```python
from build123d import *

# Parameters (mm, degrees)
SKETCH_1_W            = 101.6
SKETCH_1_H            = 101.6
EXTRUDE_1_DEPTH       = 2.9718
CUT_EXTRUDE_1_DEPTH   = 144.714827333
MIRROR_2_COPY_1_DEPTH = 144.714827333
CUT_EXTRUDE_3_DEPTH   = 144.714827333


with BuildPart() as part:
    # 草图1 → 凸台-拉伸1 (new body)
    with BuildSketch(Plane(origin=(0, 0, 0), x_dir=(1, 0, 0), z_dir=(0, 1, 0))):
        with Locations((50.8, 50.8)):
            Rectangle(SKETCH_1_W, SKETCH_1_H)
    extrude(amount=EXTRUDE_1_DEPTH)

    # 草图1<3> → 切除-拉伸1 (cut, through all)
    with BuildSketch(Plane(origin=(0, 0, 0), x_dir=(1, 0, 0), z_dir=(0, 1, 0))):
        Polygon((37.676666667, 98.6282), (37.676666667, 101.6), (30.056666667, 101.6), (30.056666667, 98.6282), (31.866666667, 98.6282), (31.866666667, 93.6282), (29.866666667, 93.6282), (29.866666667, 90.6282), (31.866666667, 90.6282), (31.866666667, 86.6282), (35.866666667, 86.6282), (35.866666667, 90.6282), (37.866666667, 90.6282), (37.866666667, 93.6282), (35.866666667, 93.6282), (35.866666667, 98.6282), align=None)
    cut_extrude_1 = extrude(amount=CUT_EXTRUDE_1_DEPTH, mode=Mode.SUBTRACT)

    # 镜向1: 切除-拉伸1 across plane
    add(cut_extrude_1.mirror(Plane(origin=(0, 0, -50.8), x_dir=(1, 0, 0), z_dir=(0, 0, -1))), mode=Mode.SUBTRACT)

    # 镜向2: 切除-拉伸1 across plane
    add(cut_extrude_1.mirror(Plane(origin=(50.8, 0, 0), x_dir=(0, 0, 1), z_dir=(1, 0, 0))), mode=Mode.SUBTRACT)

    # 镜向2 copy 1 sketch → 镜向2 copy 1 (cut, through all)
    with BuildSketch(Plane(origin=(101.6, 0, -101.6), x_dir=(-1, 0, 0), z_dir=(0, 1, 0))):
        Polygon((37.676666667, 98.6282), (37.676666667, 101.6), (30.056666667, 101.6), (30.056666667, 98.6282), (31.866666667, 98.6282), (31.866666667, 93.6282), (29.866666667, 93.6282), (29.866666667, 90.6282), (31.866666667, 90.6282), (31.866666667, 86.6282), (35.866666667, 86.6282), (35.866666667, 90.6282), (37.866666667, 90.6282), (37.866666667, 93.6282), (35.866666667, 93.6282), (35.866666667, 98.6282), align=None)
    extrude(amount=MIRROR_2_COPY_1_DEPTH, mode=Mode.SUBTRACT)

    # 草图1<4> → 切除-拉伸3 (cut, through all)
    with BuildSketch(Plane(origin=(0, 0, 0), x_dir=(1, 0, 0), z_dir=(0, 1, 0))):
        Polygon((0, 71.543333333), (0, 63.923333333), (2.9718, 63.923333333), (2.9718, 65.733333333), (7.9718, 65.733333333), (7.9718, 63.733333333), (10.9718, 63.733333333), (10.9718, 65.733333333), (14.9718, 65.733333333), (14.9718, 69.733333333), (10.9718, 69.733333333), (10.9718, 71.733333333), (7.9718, 71.733333333), (7.9718, 69.733333333), (2.9718, 69.733333333), (2.9718, 71.543333333), align=None)
    cut_extrude_3 = extrude(amount=CUT_EXTRUDE_3_DEPTH, mode=Mode.SUBTRACT)

    # 镜向3: 切除-拉伸3 across plane
    add(cut_extrude_3.mirror(Plane(origin=(0, 0, -50.8), x_dir=(1, 0, 0), z_dir=(0, 0, -1))), mode=Mode.SUBTRACT)


solid = part.part
```
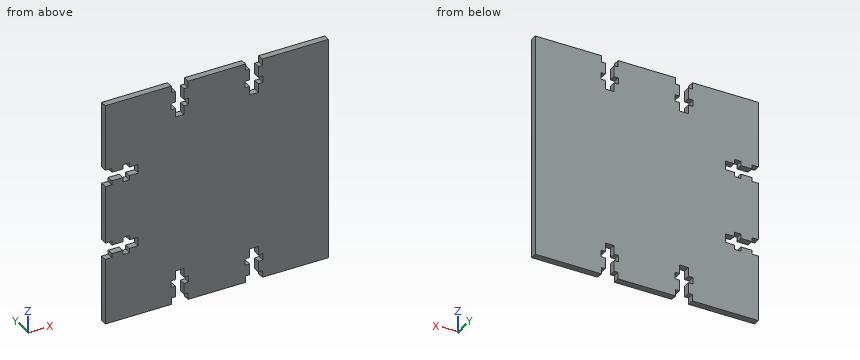
Part model, mm, in its own coordinate system. Round coordinates to 2 decimals unless told otherwise and drop trailing zeros. Order: outer loops, then holes, each group sorted by start corner. A loop starts at its lowest first (then second) coordinate and runs counter-clockwise, first axis right, second up. Notation, with made-up numbers: M -18,77 L 30,77 A12 cw 30,86 Z; hole C 4,67 d8. An arc over 180 degrees is marked long. Answer in a Markdown table with one row per item. Add a question column.
Q1. Cut at A-A on z = -68.5. Give the cut face in (x, y), and give its area (3 significant figures).
Q2. Wall check: L1, parallel to X at y = 0.7, z = -94.5; L2, parallel to X at y = 0.35, z = -71.5; L3, parallel to X at y = 1.2, z = -69. Give the ranges that are in metal, low to high. Write a range as from..to.
Q3. Pin check, flat tips, straight feed: pin 1 (0.9 mm diameter, centred on x = 37, y = 1.5, fed in from +Z); pin 2 (1.5 mm diameter, centred on x = 68, y = 1, fed in from -Z). Stop position of each tip, or through.
Established:
| question | item | result |
|---|---|---|
| 1 | outline | M 14.97,0 L 101.6,0 L 101.6,2.97 L 14.97,2.97 Z |
| 1 | area | 257 mm2 |
| 2 | L1 | x = 0..31.87, 35.87..65.73, 69.73..101.6 |
| 2 | L2 | x = 2.97..7.97, 10.97..101.6 |
| 2 | L3 | x = 14.97..101.6 |
| 3 | pin 1 | stops at z = -2.97 |
| 3 | pin 2 | stops at z = -86.63 |
